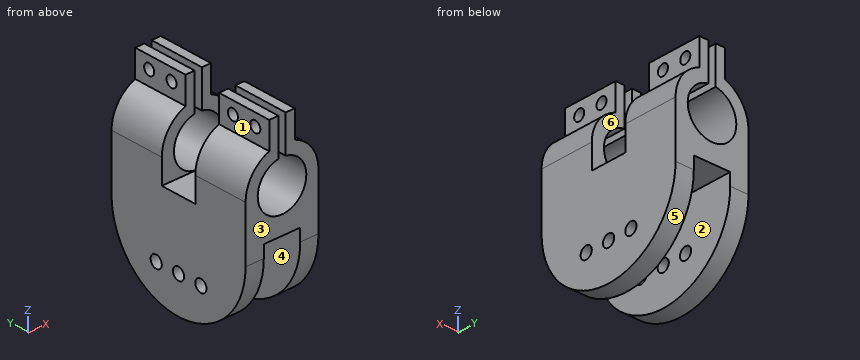
```python
from build123d import *

# Parameters (mm, degrees)
F0_R      = 30
F0_R_2    = 20
F1_DEPTH  = 120
F2_DEPTH  = 120
F4_DEPTH  = 120
F5_W      = 120
F5_H      = 30
F6_DEPTH  = 100
F7_W      = 120
F7_H      = 30
F8_DEPTH  = 50
F10_W     = 7.5
F10_H     = 45
F11_DEPTH = 25
F12_DEPTH = 25
F13_DEPTH = 25
F14_DEPTH = 25
F15_R     = 4.5
F16_DEPTH = 50
F17_R     = 4.5
F18_DEPTH = 50
F19_DEPTH = 50
F20_R     = 4.5
F21_DEPTH = 100
F22_DEPTH = 50
F23_R     = 4.5
F24_DEPTH = 50
F25_DEPTH = 100
F27_W     = 60
F27_H     = 120
F28_DEPTH = 25
F30_DEPTH = 15
F32_DEPTH = 15
F33_R     = 5
F34_DEPTH = 60.001
F35_DEPTH = 60.001
F36_DEPTH = 60.001
F37_W     = 30
F37_H     = 10
F38_DEPTH = 120.001
F39_W     = 8
F39_H     = 20
F40_DEPTH = 45
F41_DEPTH = 45
F42_W     = 8
F42_H     = 20
F43_DEPTH = 45
F44_DEPTH = 45


with BuildPart() as f1:
    # F0 (on Front) → F1 (new body)
    with BuildSketch(Plane.XZ):
        Circle(F0_R)
        Circle(F0_R_2, mode=Mode.SUBTRACT)
    extrude(amount=F1_DEPTH)

    # F0 (on Front) → F2 (join)
    with BuildSketch(Plane.XZ):
        Circle(F0_R)
        Circle(F0_R_2, mode=Mode.SUBTRACT)
    extrude(amount=F2_DEPTH)

    # F3 (on face) → F4 (cut)
    with BuildSketch(Plane.XZ.offset(120)):
        with BuildLine():
            ThreePointArc((3, 29.8496231132), (0, 30), (-3, 29.8496231132))
            Line((-3, 29.8496231132), (-3, 19.7737199333))
            ThreePointArc((-3, 19.7737199333), (0, 20), (3, 19.7737199333))
            Line((3, 19.7737199333), (3, 29.8496231132))
        make_face()
    extrude(amount=-F4_DEPTH, mode=Mode.SUBTRACT)

    # F5 (on Top) → F6 (cut)
    with BuildSketch(Plane.XY):
        with Locations((0, -60)):
            Rectangle(F5_W, F5_H)
    extrude(amount=-F6_DEPTH, mode=Mode.SUBTRACT)

    # F7 (on Top) → F8 (cut, symmetric)
    with BuildSketch(Plane.XY):
        with Locations((0, -60)):
            Rectangle(F7_W, F7_H)
    extrude(amount=F8_DEPTH, both=True, mode=Mode.SUBTRACT)

    # F17 (on face) → F18 (cut, symmetric)
    with BuildSketch(Plane.YZ.offset(10.5)):
        with Locations((-107.5, 40)):
            Circle(F17_R)
    extrude(amount=F18_DEPTH, both=True, mode=Mode.SUBTRACT)

    # F17 (on face) → F19 (cut, symmetric)
    with BuildSketch(Plane.YZ.offset(10.5)):
        with Locations((-87.5, 40)):
            Circle(F17_R)
    extrude(amount=F19_DEPTH, both=True, mode=Mode.SUBTRACT)

    # F23 (on face) → F24 (cut, symmetric)
    with BuildSketch(Plane.YZ.offset(10.5)):
        with Locations((-32.5, 40)):
            Circle(F23_R)
    extrude(amount=F24_DEPTH, both=True, mode=Mode.SUBTRACT)

    # F23 (on face) → F25 (cut)
    with BuildSketch(Plane.YZ.offset(10.5)):
        with Locations((-12.5, 40)):
            Circle(F23_R)
    extrude(amount=-F25_DEPTH, mode=Mode.SUBTRACT)



with BuildPart() as f11:
    # F10 (on offset) → F11 (new body)
    with BuildSketch(Plane.XY.offset(25)):
        with Locations((6.75, -22.5)):
            Rectangle(F10_W, F10_H)
    extrude(amount=F11_DEPTH)


with BuildPart() as f12:
    # F10 (on offset) → F12 (new body)
    with BuildSketch(Plane.XY.offset(25)):
        with Locations((-6.75, -22.5)):
            Rectangle(F10_W, F10_H)
    extrude(amount=F12_DEPTH)


with BuildPart() as f13:
    # F10 (on offset) → F13 (new body)
    with BuildSketch(Plane.XY.offset(25)):
        with Locations((-6.75, -97.5)):
            Rectangle(F10_W, F10_H)
    extrude(amount=F13_DEPTH)


with BuildPart() as f14:
    # F10 (on offset) → F14 (new body)
    with BuildSketch(Plane.XY.offset(25)):
        with Locations((6.75, -97.5)):
            Rectangle(F10_W, F10_H)
    extrude(amount=F14_DEPTH)


with BuildPart() as f16_tool:
    # F15 (on face) → F16 (new body, symmetric)
    with BuildSketch(Plane(origin=(-10.5, 0, 0), x_dir=(0, -1, 0), z_dir=(-1, 0, 0))):
        with Locations((107.5, 40)):
            Circle(F15_R)
        with Locations((87.5, 40)):
            Circle(F15_R)
    extrude(amount=F16_DEPTH, both=True)


with BuildPart() as f13_1:
    add(f13.part)

    # F16: cut by f16_tool
    add(f16_tool.part, mode=Mode.SUBTRACT)


with BuildPart() as f14_1:
    add(f14.part)

    # F16: cut by f16_tool
    add(f16_tool.part, mode=Mode.SUBTRACT)


with BuildPart() as f21_tool:
    # F20 (on face) → F21 (new body)
    with BuildSketch(Plane(origin=(-10.5, 0, 0), x_dir=(0, -1, 0), z_dir=(-1, 0, 0))):
        with Locations((12.5, 40)):
            Circle(F20_R)
    extrude(amount=-F21_DEPTH)


with BuildPart() as f11_1:
    add(f11.part)

    # F21: cut by f21_tool
    add(f21_tool.part, mode=Mode.SUBTRACT)


with BuildPart() as f12_1:
    add(f12.part)

    # F21: cut by f21_tool
    add(f21_tool.part, mode=Mode.SUBTRACT)


with BuildPart() as f22_tool:
    # F20 (on face) → F22 (new body, symmetric)
    with BuildSketch(Plane(origin=(-10.5, 0, 0), x_dir=(0, -1, 0), z_dir=(-1, 0, 0))):
        with Locations((32.5, 40)):
            Circle(F20_R)
    extrude(amount=F22_DEPTH, both=True)


with BuildPart() as f11_2:
    add(f11_1.part)

    # F22: cut by f22_tool
    add(f22_tool.part, mode=Mode.SUBTRACT)


with BuildPart() as f12_2:
    add(f12_1.part)

    # F22: cut by f22_tool
    add(f22_tool.part, mode=Mode.SUBTRACT)


with BuildPart() as f28:
    # F27 (on offset) → F28 (new body)
    with BuildSketch(Plane.XY.offset(-20)):
        with Locations((0, -60)):
            Rectangle(F27_W, F27_H)
    extrude(amount=-F28_DEPTH)

    # F29 (on face) → F30 (join)
    with BuildSketch(Plane.YZ.offset(30)):
        with BuildLine():
            Line((0, -45), (-120, -45))
            ThreePointArc((-120, -45), (-60, -105), (0, -45))
        make_face()
    extrude(amount=-F30_DEPTH)

    # F31 (on face) → F32 (join)
    with BuildSketch(Plane(origin=(-30, 0, 0), x_dir=(0, -1, 0), z_dir=(-1, 0, 0))):
        with BuildLine():
            Line((120, -45), (0, -45))
            ThreePointArc((0, -45), (60, -105), (120, -45))
        make_face()
    extrude(amount=-F32_DEPTH)

    # F33 (on face) → F34 (cut, through all)
    with BuildSketch(Plane(origin=(-30, 0, 0), x_dir=(0, -1, 0), z_dir=(-1, 0, 0))):
        with Locations((40, -75)):
            Circle(F33_R)
    extrude(amount=-F34_DEPTH, mode=Mode.SUBTRACT)

    # F33 (on face) → F35 (cut, through all)
    with BuildSketch(Plane(origin=(-30, 0, 0), x_dir=(0, -1, 0), z_dir=(-1, 0, 0))):
        with Locations((60, -75)):
            Circle(F33_R)
    extrude(amount=-F35_DEPTH, mode=Mode.SUBTRACT)

    # F33 (on face) → F36 (cut, through all)
    with BuildSketch(Plane(origin=(-30, 0, 0), x_dir=(0, -1, 0), z_dir=(-1, 0, 0))):
        with Locations((80, -75)):
            Circle(F33_R)
    extrude(amount=-F36_DEPTH, mode=Mode.SUBTRACT)

    # F37 (on face) → F38 (cut, through all)
    with BuildSketch(Plane(origin=(0, 0, 0), x_dir=(-1, 0, 0), z_dir=(0, 1, 0))):
        with Locations((0, -40)):
            Rectangle(F37_W, F37_H)
    extrude(amount=-F38_DEPTH, mode=Mode.SUBTRACT)


with BuildPart() as f40:
    # F39 (on face) → F40 (new body)
    with BuildSketch(Plane(origin=(0, 0, 0), x_dir=(-1, 0, 0), z_dir=(0, 1, 0))):
        with Locations((-26, -10)):
            Rectangle(F39_W, F39_H)
    extrude(amount=-F40_DEPTH)


with BuildPart() as f41:
    # F39 (on face) → F41 (new body)
    with BuildSketch(Plane(origin=(0, 0, 0), x_dir=(-1, 0, 0), z_dir=(0, 1, 0))):
        with Locations((26, -10)):
            Rectangle(F39_W, F39_H)
    extrude(amount=-F41_DEPTH)


with BuildPart() as f1_1:
    add(f1.part)

    add(f11_2.part)  # F43 merges F11

    add(f12_2.part)  # F43 merges F12

    add(f13_1.part)  # F43 merges F13

    add(f14_1.part)  # F43 merges F14

    add(f28.part)  # F43 merges F28

    add(f40.part)  # F43 merges F40

    add(f41.part)  # F43 merges F41
    # F42 (on face) → F43 (join)
    with BuildSketch(Plane.XZ.offset(120)):
        with Locations((-26, -10)):
            Rectangle(F42_W, F42_H)
    extrude(amount=-F43_DEPTH)

    # F42 (on face) → F44 (join)
    with BuildSketch(Plane.XZ.offset(120)):
        with Locations((26, -10)):
            Rectangle(F42_W, F42_H)
    extrude(amount=-F44_DEPTH)


solid = f1_1.part
```
CAD build for the part. Positions are in the model's coordinates, mm. Face numbers are marked on the shaded views. A direction names the side the tool comes from. Coordinates: 2 decimals unless noted, no trailing zeros. Write each loop counter-clockwise with the first axis right and the second up, starting at its lowest first coordinate (ties: lowest second). Pieces come first, ordered by that corner, then holes.
(1) Cut at D-D, the plane x = -23. List the corners of the cut face in (y, z), and give its area (3 significant figures).
(2) Cut at B-B, the plane y = -60. List the corners of the cut face in (x, z), and give its area (3 significant figures).
(3) 3-axis set-ups, long thin cutter, end or side, ignore diameter. For the marked faces 4, 5 and 6: which of +Z, -Z, +X, -X, +Y, -Y reach the whole face in a straight line?
(4) Cut at A-A, the plane x = 8. List the corners of the cut face in (y, z), and give its area (3 significant figures).
(5) Flat gauge pins, fed straight in: pin 1 (6 mm diameter, centred on y = -60, z = -75, fed in from -X); pin 2 (9 mm diameter, centred on y = -28, z = 31.5, fed in from -X); pin 3 (24 mm diameter, centred on y = -88, z = 33.5, fed in from +X); pin 4 (9 mm diameter, centred on x = -13, y = -64.5, fed in from +Z). Where does each tip first touch, or does it go through?
(6) Drill centre lines: probe 1 along X at (y, z) = (-58.5, -62); probe 2 along X at (y, z) = (-113.5, -17); probe 3 along Z at (x, y) = (-6, -107). Where is each one in solid material? Low to high.
(7) Cut at C-C, the plane z = -54. List the corners of the cut face in (x, y), and give its area (3 significant figures).
(8) Two-plate mould, pull along X, no slides. Class the marked faces 1, 2 and 3: +X half, -X half, draft (parallel to the pull), parting line (faces both ways), or undercut.
Geometry says:
1. outline: (-120, -45) arc R60 ccw to (0, -45) - (0, 19.26) - (-45, 19.26) - (-45, -20) - (-75, -20) - (-75, 19.26) - (-120, 19.26) - close; hole circle Ø10 at (-80, -75); hole circle Ø10 at (-60, -75); hole circle Ø10 at (-40, -75)
1. area: 12,000 mm2
2. outline: (-30, -105) - (-15, -105) - (-15, -80) - (-30, -80) - close; (-30, -70) - (-15, -70) - (-15, -35) - (15, -35) - (15, -70) - (30, -70) - (30, -20) - (-30, -20) - close; (15, -105) - (30, -105) - (30, -80) - (15, -80) - close
2. area: 2,700 mm2
3. face 4: -Z, +Y, -Y
3. face 5: -Z, +X, -X
3. face 6: +Z, +X, -X
4. outline: (-120, -35) - (0, -35) - (0, -18.33) - (-45, -18.33) - (-45, -20) - (-75, -20) - (-75, -18.33) - (-120, -18.33) - close; (-120, 18.33) - (-75, 18.33) - (-75, 50) - (-120, 50) - close; (-45, 18.33) - (0, 18.33) - (0, 50) - (-45, 50) - close; hole circle Ø9 at (-107.5, 40); hole circle Ø9 at (-87.5, 40); hole circle Ø9 at (-32.5, 40); hole circle Ø9 at (-12.5, 40)
4. area: 4,550 mm2
5. pin 1: passes through
5. pin 2: stops at x = -13.08
5. pin 3: stops at x = 20.92
5. pin 4: stops at z = -20
6. probe 1: x = -30 to -15, 15 to 30
6. probe 2: x = -30 to -10.54, 10.54 to 30
6. probe 3: z = -35 to -19.08, 19.08 to 35.53, 44.47 to 50
7. outline: (-30, -119.32) - (-15, -119.32) - (-15, -0.68) - (-30, -0.68) - close; (15, -119.32) - (30, -119.32) - (30, -0.68) - (15, -0.68) - close
7. area: 3,560 mm2
8. face 1: -X half
8. face 2: undercut
8. face 3: draft
